```python
from build123d import *

# Parameters (mm, degrees)
SKETCH5_R           = 3
SKETCH5_W           = 20
SKETCH5_H           = 5
SKETCH5_W_2         = 12.659523363
SKETCH5_H_2         = 7.033068536
BOSS_EXTRUDE1_DEPTH = 5
SKETCH6_W           = 330
SKETCH6_H           = 15
BOSS_EXTRUDE2_DEPTH = 5
SKETCH8_R           = 2
SKETCH8_R_2         = 3.1
CUT_EXTRUDE1_DEPTH  = 5
SKETCH9_W           = 27
SKETCH9_H           = 12
BOSS_EXTRUDE3_DEPTH = 5
SKETCH10_W          = 3.217546145
SKETCH10_H          = 2.890079535
SKETCH10_W_2        = 3.782453855
SKETCH10_H_2        = 3.521306538
SKETCH10_W_3        = 3.332881198
BOSS_EXTRUDE4_DEPTH = 30
BOSS_EXTRUDE6_DEPTH = 5
CUT_EXTRUDE4_DEPTH  = 14.3
SKETCH15_W          = 3.332881198
SKETCH15_H          = 3.521306538
SKETCH15_W_2        = 3.782453855
BOSS_EXTRUDE9_DEPTH = 14.3


with BuildPart() as part:
    # Sketch5 → Boss-Extrude1 (new body)
    with BuildSketch(Plane(origin=(0, 0, 0), x_dir=(0, 0, -1), z_dir=(1, 0, 0))):
        with BuildLine():
            Line((-40, -10), (0, -10))
            Line((0, -10), (0, 0))
            Line((0, 0), (0, 10))
            Line((0, 10), (5, 10))
            Line((5, 10), (5, 0))
            Line((5, 0), (5, -10))
            Line((5, -10), (245, -10))
            Line((245, -10), (245, 0))
            Line((245, 0), (245, 10))
            Line((245, 10), (250, 10))
            Line((250, 10), (250, 0))
            Line((250, 0), (250, -10))
            Line((250, -10), (290, -10))
            Line((290, -10), (290, 50))
            Line((290, 50), (-7.797224701, 50))
            Line((-7.797224701, 50), (-7.797224701, 69.428123594))
            ThreePointArc((-7.797224701, 69.428123594), (-10.726156889, 76.499191405), (-17.797224701, 79.428123594))
            Line((-17.797224701, 79.428123594), (-30, 79.428123594))
            ThreePointArc((-30, 79.428123594), (-37.071067812, 76.499191405), (-40, 69.428123594))
            Line((-40, 69.428123594), (-40, 50))
            Line((-40, 50), (-40, -10))
        make_face()
        with Locations((-25, 35)):
            Circle(SKETCH5_R, mode=Mode.SUBTRACT)
        with Locations((275, 35)):
            Circle(SKETCH5_R, mode=Mode.SUBTRACT)
        with Locations((89.606343961, 41.844097949)):
            Rectangle(SKETCH5_W, SKETCH5_H, mode=Mode.SUBTRACT)
        with Locations((14.606343961, 41.844097949)):
            Rectangle(SKETCH5_W, SKETCH5_H, mode=Mode.SUBTRACT)
        with Locations((-23.96746302, 63.333382994)):
            Rectangle(SKETCH5_W_2, SKETCH5_H_2, mode=Mode.SUBTRACT)
        with Locations((164.606343961, 41.844097949)):
            Rectangle(SKETCH5_W, SKETCH5_H, mode=Mode.SUBTRACT)
        with Locations((239.606343961, 41.844097949)):
            Rectangle(SKETCH5_W, SKETCH5_H, mode=Mode.SUBTRACT)
    extrude(amount=BOSS_EXTRUDE1_DEPTH)

    # Sketch6 → Boss-Extrude2 (add)
    with BuildSketch(Plane(origin=(5, 0, 0), x_dir=(0, 0, -1), z_dir=(1, 0, 0))):
        with Locations((125, -17.5)):
            Rectangle(SKETCH6_W, SKETCH6_H)
    extrude(amount=-BOSS_EXTRUDE2_DEPTH)

    # Sketch8 → Cut-Extrude1 (cut)
    with BuildSketch(Plane(origin=(5, 0, 0), x_dir=(0, 0, -1), z_dir=(1, 0, 0))):
        with Locations((30.968640194, 16)):
            Circle(SKETCH8_R)
        with Locations((30.968640194, -20)):
            Circle(SKETCH8_R)
        with Locations(Location((66.968640194, -20, 0), (0, 0, 180))):
            Circle(SKETCH8_R)
        with Locations(Location((66.968640194, 16, 0), (0, 0, 180))):
            Circle(SKETCH8_R)
        with Locations((48.968640194, -2)):
            Circle(SKETCH8_R_2)
    extrude(amount=-CUT_EXTRUDE1_DEPTH, mode=Mode.SUBTRACT)

    # Sketch9 → Boss-Extrude3 (add)
    with BuildSketch(Plane(origin=(5, 0, 0), x_dir=(0, 0, -1), z_dir=(1, 0, 0))):
        with Locations((128.106343961, 56)):
            Rectangle(SKETCH9_W, SKETCH9_H)
        Polygon((121.079302135, 59.109920465), (122.421377926, 57.767844673), (124.280039233, 57.767844673), (125.622115024, 59.109920465), (137.823890106, 59.109920465), (137.823890106, 54.109920465), (125.622115024, 54.109920465), (124.280039233, 55.451996257), (122.421377926, 55.451996257), (121.079302135, 54.109920465), (117.823890106, 54.109920465), (117.823890106, 59.109920465), align=None, mode=Mode.SUBTRACT)
    extrude(amount=-BOSS_EXTRUDE3_DEPTH)

    # Sketch10 → Boss-Extrude4 (add)
    with BuildSketch(Plane(origin=(5, 0, 0), x_dir=(0, 0, -1), z_dir=(1, 0, 0))):
        with Locations((116.215117034, 60.554960233)):
            Rectangle(SKETCH10_W, SKETCH10_H)
        with Locations((139.715117034, 60.554960233)):
            Rectangle(SKETCH10_W_2, SKETCH10_H)
        with Locations((139.715117034, 48.239346731)):
            Rectangle(SKETCH10_W_2, SKETCH10_H_2)
        with Locations((116.27278456, 48.239346731)):
            Rectangle(SKETCH10_W_3, SKETCH10_H_2)
    extrude(amount=BOSS_EXTRUDE4_DEPTH)

    # Sketch13 → Boss-Extrude6 (add)
    with BuildSketch(Plane(origin=(35, 0, 0), x_dir=(0, 0, -1), z_dir=(1, 0, 0))):
        Polygon((114.606343961, 46.478693462), (141.606343961, 46.478693462), (141.606343961, 62), (117.823890106, 62), (114.606343961, 62), align=None)
        Polygon((117.823890106, 54.109920465), (121.079302135, 54.109920465), (122.421377926, 55.451996257), (124.280039233, 55.451996257), (125.622115024, 54.109920465), (137.823890106, 54.109920465), (137.823890106, 59.109920465), (125.622115024, 59.109920465), (124.280039233, 57.767844673), (122.421377926, 57.767844673), (121.079302135, 59.109920465), (117.823890106, 59.109920465), align=None, mode=Mode.SUBTRACT)
    extrude(amount=BOSS_EXTRUDE6_DEPTH)

    # Sketch14 → Cut-Extrude4 (cut)
    with BuildSketch(Plane.ZY):
        with BuildLine():
            Line((-141.606343961, 50), (-114.606343961, 50))
            Line((-114.606343961, 50), (7.797224701, 50))
            Line((7.797224701, 50), (7.797224701, 69.428123594))
            ThreePointArc((7.797224701, 69.428123594), (10.726156889, 76.499191405), (17.797224701, 79.428123594))
            Line((17.797224701, 79.428123594), (30, 79.428123594))
            ThreePointArc((30, 79.428123594), (37.071067812, 76.499191405), (40, 69.428123594))
            Line((40, 69.428123594), (40, -25))
            Line((40, -25), (-290, -25))
            Line((-290, -25), (-290, 50))
            Line((-290, 50), (-141.606343961, 50))
        make_face()
    extrude(amount=-CUT_EXTRUDE4_DEPTH, mode=Mode.SUBTRACT)

    # Sketch15 → Boss-Extrude9 (add)
    with BuildSketch(Plane.ZY.offset(-14.3)):
        with Locations((-116.27278456, 48.239346731)):
            Rectangle(SKETCH15_W, SKETCH15_H)
        with Locations((-139.715117034, 48.239346731)):
            Rectangle(SKETCH15_W_2, SKETCH15_H)
    extrude(amount=BOSS_EXTRUDE9_DEPTH)


solid = part.part
```
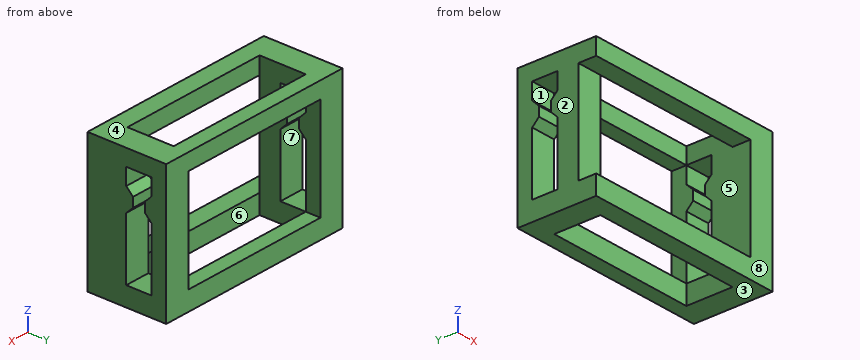
The listing builds one solid part. Answer for the finished solid, in the listing's coordinates (mm). Face numbers are marked on the shaded views. A direction names the side the tool comes from. Give positions to 0.01 mm unless a question says otherwise; leave off trailing zeros. Write each loop counter-clockwise with the first axis right and the second up, starting at its lowest first coordinate (ties: lowest second). Pieces come first, ordered by that corner, then holes. Notation, with made-up numbers: (-20, 86) -> (-13, 86) arc R28 cw to (-13, 122) -> close; hole circle Ø11 at (4.5, -14.5). An arc over 180 degrees is marked (long way). Use one line per item in the form item = value.
1) Section D-D on y = 59.75 is taken. Write down the section's boundary in (x, z).
Result:
outline = (0, -141.61) -> (40, -141.61) -> (40, -114.61) -> (0, -114.61) -> close; hole (5, -137.82) -> (35, -137.82) -> (35, -117.82) -> (5, -117.82) -> close
2) Section C-C on x = 22.5 is taken. Write down the section's boundary in (y, z), plus the area to 3 significant figures.
Result:
outline = (46.48, -141.61) -> (50, -141.61) -> (50, -137.82) -> (46.48, -137.82) -> close; (46.48, -117.94) -> (50, -117.94) -> (50, -114.61) -> (46.48, -114.61) -> close; (59.11, -141.61) -> (62, -141.61) -> (62, -137.82) -> (59.11, -137.82) -> close; (59.11, -117.82) -> (62, -117.82) -> (62, -114.61) -> (59.11, -114.61) -> close
area = 45.3 mm²
3) Straight lines are drawn through the part: probe 1 along X at (y, z) = (59.5, -134); probe 2 along Z at (x, y) = (18.5, 48.75); probe 3 along Y at (x, z) = (36, -130.5). For each, find the intervals that lie inside material, in ascending order.
Result:
probe_1 = 0 to 5, 35 to 40
probe_2 = -141.61 to -137.82, -117.94 to -114.61
probe_3 = 46.48 to 54.11, 59.11 to 62
4) Section A-A on y = 51.5 is taken. Write down the section's boundary in (x, z).
Result:
outline = (0, -141.61) -> (5, -141.61) -> (5, -114.61) -> (0, -114.61) -> close; (35, -141.61) -> (40, -141.61) -> (40, -114.61) -> (35, -114.61) -> close
5) For a pull along Z with two mould halves and no side action, classify the marked faces 1, 2, 3 and 4 as +Z half, -Z half, draft (parallel to the pull), parting line (faces both ways), or undercut.
Result:
face_1 = undercut
face_2 = draft
face_3 = -Z half
face_4 = +Z half
6) This flat-tipped pin is pushed along its axis until it touches: P1, Ø2.5, axis at x = 3.5, z = -128.5, coming from the -Y side. Where does it stop, or does it pass through?
Result:
P1 = 50
7) Section B-B on z = -132 is taken. Write down the section's boundary in (x, y).
Result:
outline = (0, 50) -> (5, 50) -> (5, 54.11) -> (0, 54.11) -> close; (0, 59.11) -> (5, 59.11) -> (5, 62) -> (0, 62) -> close; (35, 46.48) -> (40, 46.48) -> (40, 54.11) -> (35, 54.11) -> close; (35, 59.11) -> (40, 59.11) -> (40, 62) -> (35, 62) -> close
8) A tool of negligible diameter and unlimited length cuts with its end or side. For the marked faces 5, 6, 7 and 8, from which of +Z, -Z, +X, -X, +Y, -Y can it reach the whole face along a straight path? Write none if from no direction.
Result:
face_5 = none
face_6 = +Z, -Z
face_7 = +X, -X
face_8 = +Z, -Z, +X, -X, -Y
